Answer from the drawing. Dimensions are ordinates in mm from the lowest x, y and z of the part. Round coordinates to 2 decimals unless told otherwise and drop trailing zeros. Write each loop counter-clockwise with the first axis right and the second up, starting at its lowest first coordinate (ties: lowest second). Pieces come first, ordered by that corner, then holes. Notation, with made-up numbers: (-28, 60.25) - (-10, 60.25) arc R8 cw to (-10, 67.25) - close; hole circle Ø10 at (-33.5, 71.5). An arc over 180 degrees is marked (long way). One line per item, written item: value. Start each with the question number.
(1) Find the intervals of material crossed by L1, parallel to Y at x = 22, z = 43; L2, parallel to Z at x = 38, y = 50; L3, parallel to Y at x = 14, z = 72.5, in increasing order.
(2) The mould has two halves that part along Y. Classify the marked faces 1, 2 and 3: +Y half, -Y half, draft (parallel to the pull), parting line (faces both ways), or undercut.
(3) A cutting plane is placed at B-B, the plane x = 34. State how many separate pieces and enclosed holes the cut face has, plus the area to 3 significant figures.
(4) A cutting plane is placed at C-C, the plane z = 35. Determine the outline of the cut face in (x, y), plus the area to 3 significant figures.
(5) Flat-ended cylindrical pins translate along their axes: pin 1 Ø5 at (x, z) = (41.5, 78.5) entering from +Y; pin 2 Ø12 at (x, z) = (30, 36.5) entering from -Y. Find the tip coordinate at first contact, or state that the pin passes through.
(6) A cutting plane is placed at D-D, the plane z = 18. Determine the outline of the cut face in (x, y).
(7) A cutting plane is placed at A-A, the plane y = 243. Determine the outline of the cut face in (x, z).
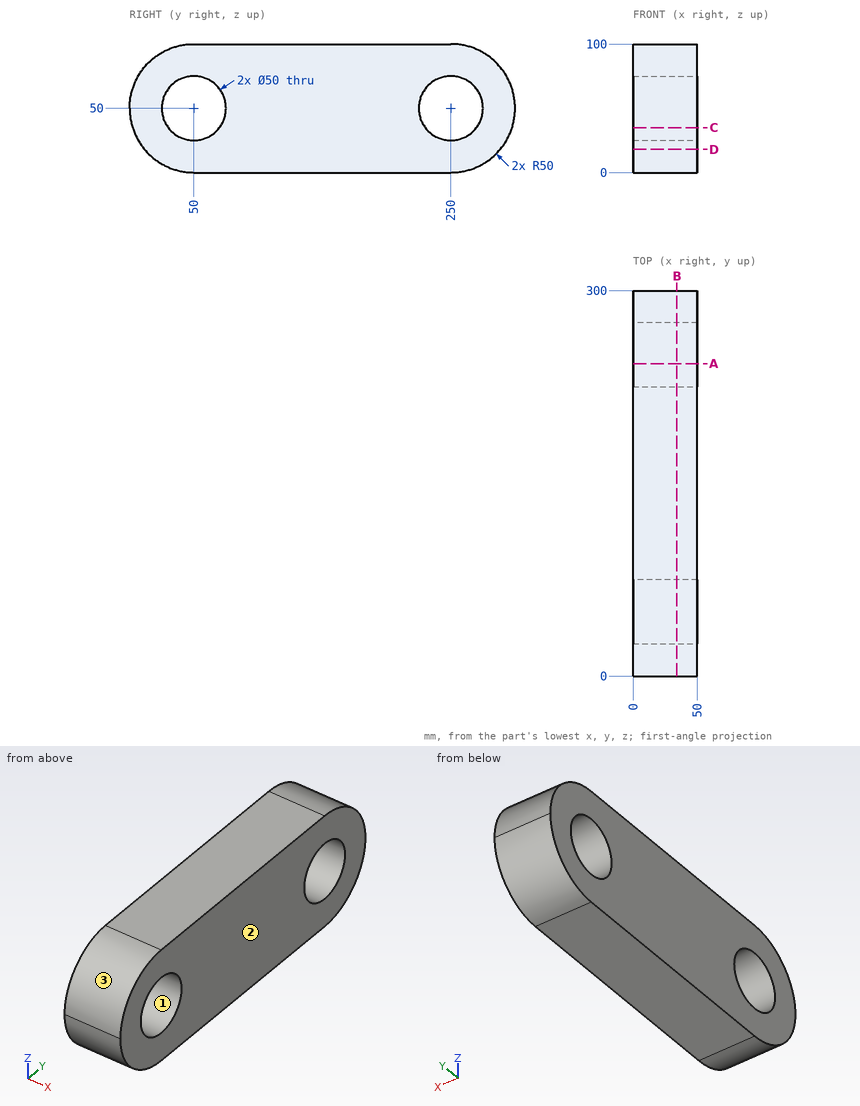
Here are the results:
1. L1: 0.49 to 26, 74 to 226, 274 to 299.51
1. L2: 0 to 25, 75 to 100
1. L3: 5.35 to 39.1, 60.9 to 239.1, 260.9 to 294.65
2. face 1: undercut
2. face 2: draft
2. face 3: -Y half
3. separate pieces: 1
3. enclosed holes: 2
3. area: 23,900 mm²
4. outline: (0, 2.3) - (50, 2.3) - (50, 30) - (0, 30) - close; (0, 70) - (50, 70) - (50, 230) - (0, 230) - close; (0, 270) - (50, 270) - (50, 297.7) - (0, 297.7) - close
4. area: 10,800 mm²
5. pin 1: y = 292.71
5. pin 2: y = 0.57
6. outline: (0, 11.58) - (50, 11.58) - (50, 288.42) - (0, 288.42) - close
7. outline: (0, 0) - (50, 0) - (50, 26) - (0, 26) - close; (0, 74) - (50, 74) - (50, 100) - (0, 100) - close
